Check sheet for the modelled part. Datum: model origin and axes. Units: mm. A direction names the side the tool comes from. Round coordinates to 2 decimals unless told otherwise and drop trailing zeros. Order: outer loops, then holes, each group sorted by start corner. A loop starts at its lowest first (then second) coordinate and runs counter-clockwise, first axis right, second up. Notation, with made-up numbers: (68, 17) -> (127, 17) arc R12 ccw to (127, 40) -> close; hole circle Ø6 at (31.5, 20.5). An arc over 180 degrees is marked (long way). Answer in a Markdown table with one row per item. Add a question column.
1. Sectioned sample at B-B, the plane y = -81. Record the boundary of the cut face in (x, z), then the cut area to 3 significant figures.
2. Access from +Z, -Z, +X, -X, +Y, -Y to the whole of each face (thin tool, end or side, straight path). Record for faces 1 (the flat face through (-31, 3, 0)), 2 (the cylindrical face through (-37.82, -26.68, 2.58)), 3 (the flat face through (-31, -66, 2.54)), 4 (the cylindrical face through (-63.842, 13.545, 20.107)).
3. Sectioned sample at D-D, the plane z = 10. Record the boundary of the cut face in (x, y).
4. Depth check by flat-ended pin: P1, Ø1.5, axis at y = -48.5, z = 1.5, coming from the +X side; P2, Ø2, axis at y = -59, z = 3.5, coming from the +X side; P3, Ø4, axis at x = -20.5, z = 22, coming from the +Y side. Enter the tip coordinate at first touch or a pass-through.
5. Sectioned sample at C-C, the plane x = -46. Record the boundary of the cut face in (y, z), then the cut area to 3 significant figures.
6. Sectioned sample at A-A, the plane y = -54.5. Record the boundary of the cut face in (x, z).
7. Draft check along X on faces 5 (the flat face through (-28, -11, 5.08)), 6 (the flat face through (-39.311, -48, 3)), 7 (the flat face through (-47.314, -60.606, 2.504)). Enter one of: +X half, -X half, draft (parallel to the pull), parting line (faces both ways), or undercut.
8. Material ranges on L1, parallel to X at y = -59, z = 3; L2, parallel to Z at x = -71, y = 44; L3, parallel to Z at x = -29, y = -42.5, recorded low to high. Write a range as from..to.
```python
from build123d import *

# Parameters (mm, degrees)
BOSS_EXTRUDE1_DEPTH = 5.08
SKETCH4_W           = 7.497155508
SKETCH4_H           = 76.250815091
CUT_EXTRUDE3_DEPTH  = 2.54
CUT_EXTRUDE4_DEPTH  = 5.08
SKETCH11_R          = 34.29
BOSS_EXTRUDE3_DEPTH = 30.48


with BuildPart() as part:
    # Sketch1 → Boss-Extrude1 (new body)
    with BuildSketch(Plane.XY):
        with BuildLine():
            Line((-26.055152411, -104.455615698), (-36.215152411, -104.455615698))
            Line((-36.215152411, -104.455615698), (-41.295152411, -104.455615698))
            Line((-41.295152411, -104.455615698), (-53.504081842, -15.511778924))
            ThreePointArc((-53.504081842, -15.511778924), (-31.135152411, 69.114610814), (-8.76622298, -15.511778924))
            Line((-8.76622298, -15.511778924), (-20.975152411, -104.455615698))
            Line((-20.975152411, -104.455615698), (-26.055152411, -104.455615698))
        make_face()
    extrude(amount=BOSS_EXTRUDE1_DEPTH)

    # Sketch4 → Cut-Extrude3 (cut)
    with BuildSketch(Plane.XY.offset(5.08)):
        with Locations((-31.244121472, -66.330208153)):
            Rectangle(SKETCH4_W, SKETCH4_H)
    extrude(amount=-CUT_EXTRUDE3_DEPTH, mode=Mode.SUBTRACT)

    # Sketch5 → Cut-Extrude4 (cut)
    with BuildSketch(Plane.XY.offset(5.08)):
        with BuildLine():
            Line((-36.262699226, -28.204800607), (-36.262699226, -67.040609222))
            ThreePointArc((-36.262699226, -67.040609222), (-37.786699226, -68.564609222), (-39.310699226, -67.040609222))
            Line((-39.310699226, -67.040609222), (-39.310699226, -28.204800607))
            ThreePointArc((-39.310699226, -28.204800607), (-37.786699226, -26.680800607), (-36.262699226, -28.204800607))
        make_face()
        with BuildLine():
            Line((-23.177543718, -28.204800607), (-23.177543718, -66.616952793))
            ThreePointArc((-23.177543718, -66.616952793), (-24.701543718, -68.140952793), (-26.225543718, -66.616952793))
            Line((-26.225543718, -66.616952793), (-26.225543718, -28.204800607))
            ThreePointArc((-26.225543718, -28.204800607), (-24.701543718, -26.680800607), (-23.177543718, -28.204800607))
        make_face()
    extrude(amount=-CUT_EXTRUDE4_DEPTH, mode=Mode.SUBTRACT)

    # Sketch11 → Boss-Extrude3 (add)
    with BuildSketch(Plane.XY.offset(5.08)):
        with Locations(Location((-31.135152411, 23.845074516, 0), (0, 0, 180))):
            Circle(SKETCH11_R)
    extrude(amount=BOSS_EXTRUDE3_DEPTH)


solid = part.part
```
Answer key:
| question | item | result |
|---|---|---|
| 1 | outline | (-44.51, 0) -> (-17.76, 0) -> (-17.76, 5.08) -> (-27.5, 5.08) -> (-27.5, 2.54) -> (-34.99, 2.54) -> (-34.99, 5.08) -> (-44.51, 5.08) -> close |
| 1 | area | 117 mm² |
| 2 | face 1 | -Z, +X, -X, +Y, -Y |
| 2 | face 2 | +Z, -Z |
| 2 | face 3 | +Z, -Y |
| 2 | face 4 | +Z |
| 3 | outline | circle Ø68.58 at (-31.14, 23.85) |
| 4 | P1 | stops at x = -13.19 |
| 4 | P2 | stops at x = -14.6 |
| 4 | P3 | stops at y = 57.03 |
| 5 | outline | (-70.18, 0) -> (66.6, 0) -> (66.6, 5.08) -> (54.75, 5.08) -> (54.75, 35.56) -> (-7.06, 35.56) -> (-7.06, 5.08) -> (-70.18, 5.08) -> close |
| 5 | area | 2,580 mm² |
| 6 | outline | (-48.15, 0) -> (-39.31, 0) -> (-39.31, 5.08) -> (-48.15, 5.08) -> close; (-36.26, 0) -> (-26.23, 0) -> (-26.23, 5.08) -> (-27.5, 5.08) -> (-27.5, 2.54) -> (-34.99, 2.54) -> (-34.99, 5.08) -> (-36.26, 5.08) -> close; (-23.18, 0) -> (-14.12, 0) -> (-14.12, 5.08) -> (-23.18, 5.08) -> close |
| 7 | face 5 | draft |
| 7 | face 6 | undercut |
| 7 | face 7 | -X half |
| 8 | L1 | x = -47.53..-39.31, -36.26..-34.99, -27.5..-26.23, -23.18..-14.74 |
| 8 | L2 | z = 0..5.08 |
| 8 | L3 | z = 0..2.54 |
